The listing builds one solid part. Answer for the finished solid, in the listing's coordinates (mm). Give positions to 0.01 mm unless a question says otherwise; leave off trailing zeros. Write each loop counter-clockwise with the first axis right and the second up, starting at its lowest first coordinate (ties: lowest second). Pieces come first, ordered by that corner, then holes. Notation, with made-up numbers: (39.5, 87) - (67.5, 87) arc R34 cw to (67.5, 119) - close; hole circle Ø3 at (12.5, 59.5). An arc over 180 degrees is marked (long way). One line per question, with ' | ' between items. Start each with the question number.
1. Given P1, Ø2, axis at x = 4, z = -14, coming from the -Y side (3 decimals); P2, Ø4, axis at x = -56, z = -14.5, coming from the +Y side; P3, Ø4, axis at x = -24, y = 19, coming from the +Z side, each flat-ended and moving along its own axis, determine where each tip first touches the part or whether it passes through.
2. Find the intervals of material crossed by L1, parallel to Y at x = 6, z = 7; L2, parallel to Y at x = -25.5, z = 4.5; L3, parallel to Z at x = -6, y = 12.75, in increasing order. Write a range as from..to.
3. A cutting plane is placed at A-A (z = -14.5). Determine the outline of the cut face in (x, y) (3 decimals), then the cut area to 4 significant figures.
```python
from build123d import *

# Parameters (mm, degrees)
CUCHILLA_SALIENTE_DEPTH                  = 60
CUCHILLA_SALIENTE_DEPTH_BACK             = 60
ENCAJE_CUCHILLA_LATERAL_CROQUIS_1_W      = 20
ENCAJE_CUCHILLA_LATERAL_CROQUIS_1_H      = 5
ENCAJE_CUCHILLA_LATERAL_SALIENTE_1_DEPTH = 2.2
ENCAJE_CUCHILLA_LATERAL_CROQUIS_2_W      = 20
ENCAJE_CUCHILLA_LATERAL_CROQUIS_2_H      = 2.5
ENCAJE_CUCHILLA_LATERAL_SALIENTE_2_DEPTH = 2.2
ENCAJE_CUCHILLA_LATERAL_CROQUIS_3_W      = 2.5
ENCAJE_CUCHILLA_LATERAL_CROQUIS_3_H      = 1.25
ENCAJE_CUCHILLA_LATERAL_SALIENTE_3_DEPTH = 1.25
ENCAJE_CUCHILLA_LATERAL_CROQUIS_4_W      = 2.5
ENCAJE_CUCHILLA_LATERAL_CROQUIS_4_H      = 1.25
ENCAJE_CUCHILLA_LATERAL_SALIENTE_4_DEPTH = 1.25
ENCAJE_CUCHILLA_LATERAL_CROQUIS_5_W      = 20
ENCAJE_CUCHILLA_LATERAL_CROQUIS_5_H      = 5
ENCAJE_CUCHILLA_LATERAL_SALIENTE_5_DEPTH = 2.2
ENCAJE_CUCHILLA_LATERAL_CROQUIS_6_W      = 20
ENCAJE_CUCHILLA_LATERAL_CROQUIS_6_H      = 2.5
ENCAJE_CUCHILLA_LATERAL_SALIENTE_6_DEPTH = 2.2
ENCAJE_CUCHILLA_LATERAL_CROQUIS_7_W      = 2.5
ENCAJE_CUCHILLA_LATERAL_CROQUIS_7_H      = 1.25
ENCAJE_CUCHILLA_LATERAL_SALIENTE_7_DEPTH = 1.25
ENCAJE_CUCHILLA_LATERAL_CROQUIS_8_W      = 2.5
ENCAJE_CUCHILLA_LATERAL_CROQUIS_8_H      = 1.25
ENCAJE_CUCHILLA_LATERAL_SALIENTE_8_DEPTH = 1.25
ENCAJE_CUCHILLA_CENTRAL_SALIENTE_DEPTH   = 20


with BuildPart() as part:
    # Croquis4 → Cuchilla-Saliente (new, two sides: drawn at the far end of the back side and taken through both)
    with BuildSketch(Plane(origin=(0, 0, 0), x_dir=(0, 0, -1), z_dir=(1, 0, 0)).offset(-CUCHILLA_SALIENTE_DEPTH_BACK)):
        with BuildLine():
            Line((9.97060468, 23.467626264), (7.47060468, 23.467626264))
            add(Edge.make_bspline(
                [(-15, 1), (0.62292895, 1), (7.47060468, 23.467626264)],
                knots=[0, 0, 0, 1.117079483, 1.117079483, 1.117079483], degree=2, weights=[1, 0.848029877, 1]))
            Line((-15, 1), (-17, 0))
            Line((-17, 0), (0, 0))
            Line((0, 0), (0, 5))
            add(Edge.make_bspline(
                [(0, 5), (9.261036245, 5), (9.97060468, 23.467626264)],
                knots=[0, 0, 0, 1.494102477, 1.494102477, 1.494102477], degree=2, weights=[1, 0.733695675, 1]))
        make_face()
    extrude(amount=CUCHILLA_SALIENTE_DEPTH + CUCHILLA_SALIENTE_DEPTH_BACK)

    # Encaje-Cuchilla-Lateral-Croquis-1 → Encaje-Cuchilla-Lateral-Saliente-1 (add)
    with BuildSketch(Plane(origin=(60, 0, 0), x_dir=(0, 0, -1), z_dir=(1, 0, 0))):
        with Locations((10, 2.5)):
            Rectangle(ENCAJE_CUCHILLA_LATERAL_CROQUIS_1_W, ENCAJE_CUCHILLA_LATERAL_CROQUIS_1_H)
    extrude(amount=-ENCAJE_CUCHILLA_LATERAL_SALIENTE_1_DEPTH)

    # Encaje-Cuchilla-Lateral-Croquis-2 → Encaje-Cuchilla-Lateral-Saliente-2 (add)
    with BuildSketch(Plane.ZY.offset(-57.8)):
        with Locations((-10, 1.25)):
            Rectangle(ENCAJE_CUCHILLA_LATERAL_CROQUIS_2_W, ENCAJE_CUCHILLA_LATERAL_CROQUIS_2_H)
    extrude(amount=ENCAJE_CUCHILLA_LATERAL_SALIENTE_2_DEPTH)

    # Encaje-Cuchilla-Lateral-Croquis-3 → Encaje-Cuchilla-Lateral-Saliente-3 (add)
    with BuildSketch(Plane.ZY.offset(-55.6)):
        with Locations((-18.75, 1.875)):
            Rectangle(ENCAJE_CUCHILLA_LATERAL_CROQUIS_3_W, ENCAJE_CUCHILLA_LATERAL_CROQUIS_3_H)
    extrude(amount=ENCAJE_CUCHILLA_LATERAL_SALIENTE_3_DEPTH)

    # Encaje-Cuchilla-Lateral-Croquis-4 → Encaje-Cuchilla-Lateral-Saliente-4 (add)
    with BuildSketch(Plane.ZY.offset(-57.8)):
        with Locations((-18.75, 4.375)):
            Rectangle(ENCAJE_CUCHILLA_LATERAL_CROQUIS_4_W, ENCAJE_CUCHILLA_LATERAL_CROQUIS_4_H)
    extrude(amount=ENCAJE_CUCHILLA_LATERAL_SALIENTE_4_DEPTH)



with BuildPart() as body_2:
    # Encaje-Cuchilla-Lateral-Croquis-5 → Encaje-Cuchilla-Lateral-Saliente-5 (new body)
    with BuildSketch(Plane.ZY.offset(60)):
        with Locations((-10, 2.5)):
            Rectangle(ENCAJE_CUCHILLA_LATERAL_CROQUIS_5_W, ENCAJE_CUCHILLA_LATERAL_CROQUIS_5_H)
    extrude(amount=-ENCAJE_CUCHILLA_LATERAL_SALIENTE_5_DEPTH)


with BuildPart() as part_1:
    add(part.part)

    add(body_2.part)  # Encaje-Cuchilla-Lateral-Saliente-6 merges body 2
    # Encaje-Cuchilla-Lateral-Croquis-6 → Encaje-Cuchilla-Lateral-Saliente-6 (add)
    with BuildSketch(Plane(origin=(-57.8, 0, 0), x_dir=(0, 0, -1), z_dir=(1, 0, 0))):
        with Locations((10, 1.25)):
            Rectangle(ENCAJE_CUCHILLA_LATERAL_CROQUIS_6_W, ENCAJE_CUCHILLA_LATERAL_CROQUIS_6_H)
    extrude(amount=ENCAJE_CUCHILLA_LATERAL_SALIENTE_6_DEPTH)

    # Encaje-Cuchilla-Lateral-Croquis-7 → Encaje-Cuchilla-Lateral-Saliente-7 (add)
    with BuildSketch(Plane(origin=(-57.8, 0, 0), x_dir=(0, 0, -1), z_dir=(1, 0, 0))):
        with Locations((18.75, 4.375)):
            Rectangle(ENCAJE_CUCHILLA_LATERAL_CROQUIS_7_W, ENCAJE_CUCHILLA_LATERAL_CROQUIS_7_H)
    extrude(amount=ENCAJE_CUCHILLA_LATERAL_SALIENTE_7_DEPTH)

    # Encaje-Cuchilla-Lateral-Croquis-8 → Encaje-Cuchilla-Lateral-Saliente-8 (add)
    with BuildSketch(Plane(origin=(-55.6, 0, 0), x_dir=(0, 0, -1), z_dir=(1, 0, 0))):
        with Locations((18.75, 1.875)):
            Rectangle(ENCAJE_CUCHILLA_LATERAL_CROQUIS_8_W, ENCAJE_CUCHILLA_LATERAL_CROQUIS_8_H)
    extrude(amount=ENCAJE_CUCHILLA_LATERAL_SALIENTE_8_DEPTH)

    # Encaje-Cuchilla-Central-Croquis → Encaje-Cuchilla-Central-Saliente (add)
    with BuildSketch(Plane(origin=(0, 0, 0), x_dir=(-1, 0, 0), z_dir=(0, 0, -1))):
        Polygon((2.5, 3.125), (5, 3.125), (5, 1.875), (2.5, 1.875), (2.5, 0), (-2.5, 0), (-2.5, 1.875), (-5, 1.875), (-5, 3.125), (-2.5, 3.125), (-2.5, 5), (2.5, 5), align=None)
    extrude(amount=ENCAJE_CUCHILLA_CENTRAL_SALIENTE_DEPTH)


solid = part_1.part
```
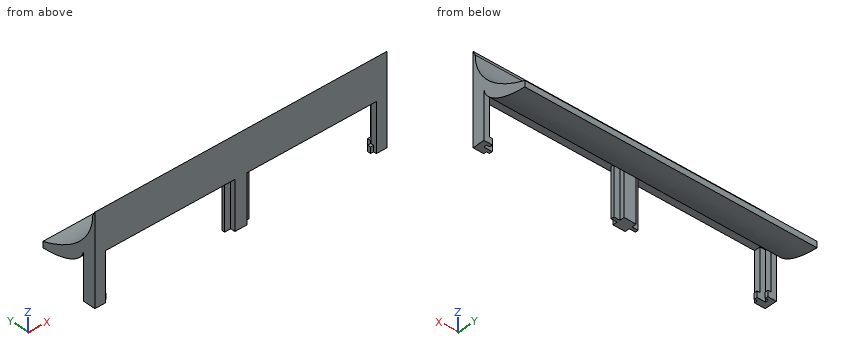
Determined:
1) P1: y = 1.875 | P2: y = 5 | P3: z = -5
2) L1: 0..3.1 | L2: 0..4.7 | L3: -7.9..-2.7
3) outline: (-60, 0) - (-55.6, 0) - (-55.6, 2.5) - (-57.8, 2.5) - (-57.8, 5) - (-60, 5) - close; (-5, 1.875) - (-2.5, 1.875) - (-2.5, 0) - (2.5, 0) - (2.5, 1.875) - (5, 1.875) - (5, 3.125) - (2.5, 3.125) - (2.5, 5) - (-2.5, 5) - (-2.5, 3.125) - (-5, 3.125) - close; (55.6, 0) - (60, 0) - (60, 5) - (57.8, 5) - (57.8, 2.5) - (55.6, 2.5) - close | area: 64.25 mm2
